from build123d import *

# Parameters (mm, degrees)
F0_W     = 101.6
F0_H     = 50.8
F1_DEPTH = 1117.6
F2_W     = 25.4
F2_H     = 101.6
F2_H_2   = 127
F3_DEPTH = 101.601
F4_R     = 3.175
F5_DEPTH = 50.801


with BuildPart() as f1:
    # F0 (on Top) → F1 (new body)
    with BuildSketch(Plane.XY):
        Rectangle(F0_W, F0_H)
    extrude(amount=F1_DEPTH)

    # F2 (on face) → F3 (cut, through all)
    with BuildSketch(Plane.YZ.offset(50.8)):
        with Locations((12.7, 457.2)):
            Rectangle(F2_W, F2_H)
        with Locations((12.7, 50.8)):
            Rectangle(F2_W, F2_H)
        with Locations((12.7, 1066.8)):
            Rectangle(F2_W, F2_H)
        with Locations((-12.7, 876.3)):
            Rectangle(F2_W, F2_H_2)
    extrude(amount=-F3_DEPTH, mode=Mode.SUBTRACT)

    # F4 (on face) → F5 (cut, through all)
    with BuildSketch(Plane.XZ.offset(25.4)):
        with Locations((-25.4, 1066.8)):
            Circle(F4_R)
        with Locations((-25.4, 457.2)):
            Circle(F4_R)
        with Locations((-25.4, 50.8)):
            Circle(F4_R)
        with Locations((25.4, 1066.8)):
            Circle(F4_R)
        with Locations((25.4, 457.2)):
            Circle(F4_R)
        with Locations((25.4, 50.8)):
            Circle(F4_R)
        with Locations((-25.4, 863.6)):
            Circle(F4_R)
        with Locations((25.4, 863.6)):
            Circle(F4_R)
    extrude(amount=-F5_DEPTH, mode=Mode.SUBTRACT)


solid = f1.part
Geometry: final body of the model. Coordinates: model frame, mm. A direction names the side the tool comes from. Give positions to 0.01 mm unless a question says otherwise; leave off trailing zeros. Write each loop counter-clockwise with the first axis right and the second up, starting at its lowest first coordinate (ties: lowest second). Pieces come first, ordered by that corner, then holes. Notation, with made-up numbers: (79, 16) -> (118, 16) arc R27 ccw to (118, 37) -> close; hole circle Ø5 at (83.25, 0). An arc over 180 degrees is marked (long way). Answer as a JSON object with one key per item and string values.
1. Cut plane B-B on x = -2.5. Output: boundary loops of the cut face in (y, z).
Ans:
{"outline": "(-25.4, 0) -> (0, 0) -> (0, 101.6) -> (25.4, 101.6) -> (25.4, 406.4) -> (0, 406.4) -> (0, 508) -> (25.4, 508) -> (25.4, 1016) -> (0, 1016) -> (0, 1117.6) -> (-25.4, 1117.6) -> (-25.4, 939.8) -> (0, 939.8) -> (0, 812.8) -> (-25.4, 812.8) -> close"}
2. Contact query for flat-ended pins moving along their axis: pin 1 (4 mm diameter, centred on x = -23, y = -8.5, fed in from -Z); pin 2 (8.5 mm diameter, centred on x = 25.4, z = 50.8, fed in from +Y); pin 3 (8.5 mm diameter, centred on x = -25.4, z = 863.6, fed in from -Y); pin 4 (20.5 mm diameter, centred on x = 15.5, y = 19, fed in from +Z). Output: stop coordinate, or through.
Ans:
{"pin 1": "stops at z = 0", "pin 2": "stops at y = 0", "pin 3": "stops at y = 0", "pin 4": "stops at z = 1016"}
3. Mould query, pull axis Z, two halves, no side actions, for faces 5 (the flat face through (1, 0, 456)), 6 (the flat face through (1, 0, 50)), 7 (the flat face through (-1, -13, 1117.6)). Classes: pulls with the +Z half, pulls with the -Z half, needs draft (parallel to the pull), parting line crosses it, or undercut.
Ans:
{"face 5": "undercut", "face 6": "needs draft", "face 7": "pulls with the +Z half"}
4. Access query for faces 1 (the flat face through (1, 13, 508)), 2 (the flat face through (1, 0, 1066)), 3 (the flat face through (1, 13, 101.6)), 4 (the flat face through (1, -13, 812.8)). Directions: +Z, -Z, +X, -X, +Y, -Y. A direction counts if a zero-diameter tool reaches every point of the face in a straight line with its end or side. Return the directions, or none.
Ans:
{"face 1": "+X, -X, +Y", "face 2": "+Z, +X, -X, +Y", "face 3": "-Z, +X, -X, +Y", "face 4": "+X, -X, -Y"}
5. Cut plane A-A on y = -11. Output: boundary loops of the cut face in (x, z) (3 decimals), and give its area (3 significant figures).
Ans:
{"outline": "(-50.8, 0) -> (50.8, 0) -> (50.8, 812.8) -> (-50.8, 812.8) -> close; (-50.8, 939.8) -> (50.8, 939.8) -> (50.8, 1117.6) -> (-50.8, 1117.6) -> close; hole circle Ø6.35 at (-25.4, 50.8); hole circle Ø6.35 at (-25.4, 457.2); hole circle Ø6.35 at (-25.4, 1066.8); hole circle Ø6.35 at (25.4, 50.8); hole circle Ø6.35 at (25.4, 457.2); hole circle Ø6.35 at (25.4, 1066.8)", "area": "100,000 mm^2"}
6. Ray query, probe 1 along Z at (x, y) = (25.4, -6.5) (3 decimals); probe 2 along X at (y, z) = (13, 863); probe 3 along X at (y, z) = (-6.75, 457.2) (3 decimals). Return the intervals inside material, ascending. Write a range as from..to.
Ans:
{"probe 1": "z = 0..47.625, 53.975..454.025, 460.375..812.8, 939.8..1063.625, 1069.975..1117.6", "probe 2": "x = -50.8..-28.52, -22.28..22.28, 28.52..50.8", "probe 3": "x = -50.8..-28.575, -22.225..22.225, 28.575..50.8"}
